Read the model definition and answer for the solid it produces. Units are mm, in the model's axes. A direction names the side the tool comes from. Give positions to 0.01 mm unless a question says otherwise; leave off trailing zeros. Order: outer loops, then holes, each group sorted by start corner. A loop starts at its lowest first (then second) coordinate and runs counter-clockwise, first axis right, second up. Notation, with made-up numbers: M -29,-16 L 8,-16 A9 cw 8,-6 Z; hole C -21.75,-16 d4. An arc over 180 degrees is marked long. One line per item, written item: value. Start each with the question number.
Autodesk Inventor part; units mm, degrees
ref_plane "YZ Plane" through (0, 0, 0) normal (1, 0, 0) x (0, 1, 0)
ref_plane "XZ Plane" through (0, 0, 0) normal (0, 1, 0) x (-1, 0, 0)
ref_plane "XY Plane" through (0, 0, 0) normal (0, 0, 1) x (1, 0, 0)
sketch "Sketch1" plane through (0, 0, 0) normal (0, 0, 1) x (1, 0, 0)
  line L0 (0, 0) -> (45, 0)
  line L1 (50, -5) -> (50, -35)
  line L2 (50, -35) -> (60, -35)
  line L3 (60, -35) -> (60, 30)
  arc A0 (60, 30) -> (30, 30) centre (45, 30) ccw
  line L4 (30, 30) -> (30, 15.6159)
  line L5 (30, 15.6159) -> (30, 15)
  arc A1 (25, 10) -> (30, 15) centre (25, 15) ccw
  line L6 (25, 10) -> (0, 10)
  line L7 (0, 10) -> (0, 0)
  arc A2 (50, -5) -> (45, 0) centre (45, -5) ccw
  circle A3 centre (45, 30) radius 5
  dimension "d0" = 5
  dimension "d1" = 10
  dimension "d2" = 30
  dimension "d3" = 10
  dimension "d4" = 10
  dimension "d5" = 60
  dimension "d6" = 35
  dimension "d7" = 65
extrude "Extrusion1" add sketch "Sketch1" along normal blind 30
fillet "Fillet1" radius 15 4 edges at (0, 5, 30) (0, 5, 0) (55, -35, 30) (55, -35, 0)
sketch "Sketch2" plane through (60, 30, 30) normal (1, 0, 0) x (0, 0, -1)
  arc A0 (0, -50) -> (30, -50) centre (15, -50) ccw
  circle A1 centre (15, -50) radius 5
  line L0 (20, 15) -> (20, -20)
  line L1 (20, -20) -> (10, -20)
  line L2 (10, -20) -> (10, 15)
  line L3 (30, 15) -> (0, 15)
  line L4 (30, 15) -> (30, 0)
  line L5 (30, -20) -> (0, -20)
  point P0 (30, -30)
  point P1 (15, -20)
  point P2 (15, 15)
  point P3 (20, 15)
  dimension "d11" = 10
  dimension "d12" = 10
extrude "Extrusion2" cut sketch "Sketch2" against normal through all
sketch "Sketch3" plane through (15, 10, 0) normal (0, 1, 0) x (1, 0, 0)
  arc A0 (0, 0) -> (0, -30) centre (0, -15) ccw
  circle A1 centre (0, -15) radius 5
  point P0 (-15, 0)
  dimension "d15" = 10
extrude "Extrusion3" cut sketch "Sketch3" against normal through all
properties part number "b5"
Q1. Find section A-A, the plane y = 36.5. Give the vertices of the cut face in (x, z), then the cut area to 3 significant figures.
Q2. Find section D-D, the plane y = -22. Give the vertices of the cut face in (x, z), then the cut area to 3 significant figures.
Q3. A tool of negligible diameter and unlimited length cuts with its end or side. For faces 5 (the flat face through (24, 10, 15)), 6 (the flat face through (47, 24, 10)), 7 (the flat face through (30, 23, 5)), from which of +Z, -Z, +X, -X, +Y, -Y can it reach the whole face along a straight path? Write none if from no direction.
Q4. Consider probe 1 along X at (y, z) = (30, 25); probe 2 along Y at (x, z) = (45, 27.75); probe 3 along Z at (x, y) = (15, 5.25). Determine where each line is inside the solid, lowest interval first.
Q5. Find section C-C, the plane z = 23.5. Give the vertices of the cut face in (x, y).
Q6. Determine the mould class of faces 1 (the cylindrical face through (55.07, -24.88, 16.08)), 2 (the cylindrical face through (48, -1, 15)), 3 (the cylindrical face through (41, 33, 25)), 4 (the flat face through (30, 23, 25)) for opening direction Y: released by +Y, released by -Y, zero draft, split by the parting line, or undercut.
Q7. Each of these flat-tipped pins is pushed along its axis until it touches: pin 1 (3 mm diameter, centred on y = 24.5, z = 7, fed in from -X); pin 2 (15 mm diameter, centred on y = -20, z = 17, fed in from -X); pin 3 (15 mm diameter, centred on x = 27.5, z = 20, fed in from -Y). Where does it stop, or does it pass through?
Evaluation:
1. outline: M 31.48,0 L 58.52,0 L 58.52,10 L 31.48,10 Z; M 31.48,20 L 58.52,20 L 58.52,30 L 31.48,30 Z
1. area: 541 mm2
2. outline: M 50,0.13 L 60,0.13 L 60,10.42 L 50,10.42 Z; M 50,19.58 L 60,19.58 L 60,29.87 L 50,29.87 Z
2. area: 206 mm2
3. face 5: -X, +Y
3. face 6: +X, -X, +Y
3. face 7: +Z, -Z, -X, +Y
4. probe 1: 30 to 40, 50 to 60
4. probe 2: 0 to 25, 35 to 45
4. probe 3: 0 to 10, 20 to 30
5. outline: M 2.64,0 L 45,0 A5 cw 50,-5 L 50,-32.36 L 60,-32.36 L 60,30 A15 ccw 30,30 L 30,15 A5 cw 25,10 L 2.64,10 Z; hole C 45,30 d10
6. face 1: undercut
6. face 2: released by -Y
6. face 3: undercut
6. face 4: zero draft
7. pin 1: x = 30
7. pin 2: x = 50
7. pin 3: y = 0
